Check sheet for the modelled part. Datum: model origin and axes. Units: mm. A direction names the side the tool comes from. Coordinates: 2 decimals unless noted, no trailing zeros. Write each loop counter-clockwise with the first axis right and the second up, starting at its lowest first coordinate (ties: lowest second). Pieces come first, ordered by that corner, then holes. Notation, with made-up numbers: M -11.5,13 L 2.5,13 A17 cw 2.5,19 Z; hole C 57.25,-33.75 d7. An arc over 180 degrees is marked long. Answer as CSV lines item,"result". Start each with the question number.
1) Section check D-D (z = 1.5). Record the cut outline in (x, y).
2) Access from +Z, -Z, +X, -X, +Y, -Y to the whole of each face (thin tool, end or side, straight path). Record for faces 1 (the flat face through (0, 18, 6)), 2 (the cylindrical face through (-9.526, -9.648, 1.972)).
3) Section check C-C (z = 5). Record the cut outline in (x, y).
4) Material ranges on L1, parallel to Y at x = -11, z = 5.8; L2, parallel to Y at x = 11, z = 1.4; L3, parallel to Y at x = 0, z = 3.5, recorded low to high. Write a range as [from, to].
5) Section check A-A (x = 0). Record the cut outline in (y, z).
6) Go/stop test with flat-tipped pins: pin 1 Ø16 at (x, y) = (0, 0) entering from +Z; pin 2 Ø2 at (x, y) = (11.5, 11.5) entering from -Z. Record where each tip stops, or that it passes through.
7) Draft check along X on faces 3 (the cylindrical face through (12.524, 10.368, 5.521)), 4 (the cylindrical face through (15.9, 16, 6.2)), 5 (the conical face through (10.85, -10.76, 7.82)), 6 (the cylindrical face through (-16, 15.9, 6.2)). Enter one of: +X half, -X half, draft (parallel to the pull), parting line (faces both ways), or undercut.
from build123d import *

# Parameters (mm, degrees)
ESBO_O1_R                       = 5
RESSALTO_EXTRUS_O1_DEPTH        = 12.5
FURO_ROSCADO_DE_M41_D           = 3.3
FURO_ROSCADO_DE_M41_DEPTH       = 7
FURO_ROSCADO_DE_M41_CBORE_D     = 4
FURO_ROSCADO_DE_M41_CBORE_DEPTH = 4
FURO_ROSCADO_DE_M41_TIP         = 0.991420021


with BuildPart() as part:
    # Esboço1 → Ressalto-extrusão1 (new body)
    with BuildSketch(Plane.XY):
        with BuildLine():
            Line((-11, 18), (11, 18))
            ThreePointArc((11, 18), (15.949747468, 15.949747468), (18, 11))
            Line((18, 11), (18, -11))
            ThreePointArc((18, -11), (15.949747468, -15.949747468), (11, -18))
            Line((11, -18), (-11, -18))
            ThreePointArc((-11, -18), (-15.949747468, -15.949747468), (-18, -11))
            Line((-18, -11), (-18, 11))
            ThreePointArc((-18, 11), (-15.949747468, 15.949747468), (-11, 18))
        make_face()
        Circle(ESBO_O1_R, mode=Mode.SUBTRACT)
    extrude(amount=RESSALTO_EXTRUS_O1_DEPTH)

    # Furo roscado de M41
    with Locations(Plane(origin=(0, 0, 0), x_dir=(-1, 0, 0), z_dir=(0, 0, -1))):
        with Locations((11, -11), (0, 0), (11, 11), (-11, -11), (-11, 11)):
            CounterBoreHole(FURO_ROSCADO_DE_M41_D / 2, FURO_ROSCADO_DE_M41_CBORE_D / 2, FURO_ROSCADO_DE_M41_CBORE_DEPTH, depth=FURO_ROSCADO_DE_M41_DEPTH)
            with Locations((0, 0, -(FURO_ROSCADO_DE_M41_DEPTH + FURO_ROSCADO_DE_M41_TIP / 2))):  # 118° drill point
                Cone(0, FURO_ROSCADO_DE_M41_D / 2, FURO_ROSCADO_DE_M41_TIP, mode=Mode.SUBTRACT)


solid = part.part
Results found:
1,outline,"M -18,-11 A7 ccw -11,-18 L 11,-18 A7 ccw 18,-11 L 18,11 A7 ccw 11,18 L -11,18 A7 ccw -18,11 Z; hole C -11,-11 d4; hole C -11,11 d4; hole C 0,0 d10; hole C 11,-11 d4; hole C 11,11 d4"
2,face 1,"+Z, -Z, +X, -X, +Y"
2,face 2,"-Z"
3,outline,"M -18,-11 A7 ccw -11,-18 L 11,-18 A7 ccw 18,-11 L 18,11 A7 ccw 11,18 L -11,18 A7 ccw -18,11 Z; hole C -11,-11 d3.3; hole C -11,11 d3.3; hole C 0,0 d10; hole C 11,-11 d3.3; hole C 11,11 d3.3"
4,L1,"y = [-18, -12.65], [-9.35, 9.35], [12.65, 18]"
4,L2,"y = [-18, -13], [-9, 9], [13, 18]"
4,L3,"y = [-18, -5], [5, 18]"
5,outline,"M -18,0 L -5,0 L -5,12.5 L -18,12.5 Z; M 5,0 L 18,0 L 18,12.5 L 5,12.5 Z"
6,pin 1,"stops at z = 12.5"
6,pin 2,"stops at z = 4"
7,face 3,"undercut"
7,face 4,"+X half"
7,face 5,"undercut"
7,face 6,"-X half"
